from build123d import *

# Parameters (mm, degrees)
CROQUIS1_W              = 56
CROQUIS1_H              = 56
CROQUIS1_R              = 2
SALIENTE_EXTRUIR2_DEPTH = 0.8
CROQUIS4_R              = 4
CROQUIS4_W              = 3.55
CROQUIS4_H              = 40
CORTAR_EXTRUIR1_DEPTH   = 10
CORTAR_EXTRUIR2_START   = -42.374993
CROQUIS7_R              = 2
CORTAR_EXTRUIR2_DEPTH   = 28.749989
SALIENTE_EXTRUIR4_DEPTH = 10


with BuildPart() as part:
    # Croquis1 → Saliente-Extruir2 (new body)
    with BuildSketch(Plane.XY):
        Rectangle(CROQUIS1_W, CROQUIS1_H)
        Circle(CROQUIS1_R, mode=Mode.SUBTRACT)
    extrude(amount=SALIENTE_EXTRUIR2_DEPTH)

    # Croquis2 → Revolución1 (revolve)
    with BuildSketch(Plane(origin=(0, 0, 0), x_dir=(0, 0, -1), z_dir=(1, 0, 0))):
        Polygon((-0.8, 0), (-10.8, 0), (-10.8, 10), (-2.8, 15), (-0.8, 15), align=None)
    revolve(axis=Axis((0, 0, 0.8), (0, 0, 1)))

    # Croquis4 → Cortar-Extruir1 (cut)
    with BuildSketch(Plane.XY.offset(10.8)):
        Circle(CROQUIS4_R)
        with Locations((-6.675, 0)):
            Rectangle(CROQUIS4_W, CROQUIS4_H)
        with Locations((6.675, 0)):
            Rectangle(CROQUIS4_W, CROQUIS4_H)
    extrude(amount=-CORTAR_EXTRUIR1_DEPTH, mode=Mode.SUBTRACT)

    # Croquis7 → Cortar-Extruir2 (cut)
    with BuildSketch(Plane.ZY.offset(28).offset(CORTAR_EXTRUIR2_START)):
        with Locations((5.8, 0)):
            Circle(CROQUIS7_R)
    extrude(amount=CORTAR_EXTRUIR2_DEPTH, mode=Mode.SUBTRACT)

    # Croquis3 → Saliente-Extruir4 (add)
    with BuildSketch(Plane.XY.offset(0.8)):
        with BuildLine():
            Line((23, -28), (28, -28))
            Line((28, -28), (28, -23))
            ThreePointArc((28, -23), (31.535533906, -31.535533906), (23, -28))
        make_face()
    extrude(amount=SALIENTE_EXTRUIR4_DEPTH)


with BuildPart() as saliente_extruir4_kept_piece:
    # of the separate pieces the step leaves, the one the design keeps (saliente_extruir4_pieces_kept)
    add(part.part.solids().sort_by_distance((28, -28, 0))[0])


solid = saliente_extruir4_kept_piece.part
Geometry check sheet. Reference: the model listing, model coordinates, mm. A direction names the side the tool comes from. Round coordinates to 2 decimals unless told otherwise and drop trailing zeros. Write each loop counter-clockwise with the first axis right and the second up, starting at its lowest first coordinate (ties: lowest second). Pieces come first, ordered by that corner, then holes. Notation, with made-up numbers: (-23, -11.5) -> (-2, -11.5) arc R14 ccw to (-2, 14.5) -> close; hole circle Ø2 at (22, -22.75). An arc over 180 degrees is marked (long way). One line per item, written item: value. Start each with the question number.
(1) Draft check along Y on faces 6 (the cylindrical face through (0, 15, 2)), 7 (the cylindrical face through (-0.434, -1.952, 0.394)), 8 (the cylindrical face through (-3.2, -2.4, 5.9)), 9 (the flat face through (-9, 0, 10.8)). Enter one of: +Y half, -Y half, draft (parallel to the pull), parting line (faces both ways), or undercut.
(2) Go/stop test with flat-tipped pins: pin 1 Ø3 at (x, y) = (0, 0) entering from -Z; pin 2 Ø1.5 at (x, y) = (22, -7) entering from +Z; pin 3 Ø4.5 at (y, z) = (0, 5.8) entering from +X; pin 4 Ø5 at (y, z) = (0, 5.8) entering from +X. Record where each tip stops, or that it passes through.
(3) Cross-section at B-B, the plane z = 8.75. Record the cut outline in (x, y).
(4) Scan lines: line 1 (X direction, y = 12, z = 1.75); line 2 (X direction, y = 8, z = 7.25); line 3 (Z direction, x = -4.15, y = 0). Record each from-to range of solid material in increasing order. Write a range as [from, to].
(5) Access from +Z, -Z, +X, -X, +Y, -Y to the whole of each face (thin tool, end or side, straight path). Record for faces 1 (the flat face through (0, 7, 0)), 2 (the cylindrical face through (-15, 0, 2)), 3 (the cylindrical face through (15, 0, 2)), 4 (the flat face through (-8.45, -0.2, 3.6)), 5 (the flat face through (-2, -1, 0.8)).
(6) Cross-section at A-A, the plane x = 0. Record the cut outline in (y, z), and give its area (3 significant figures).
(7) Cross-section at D-D, the plane y = 21. Record the cut outline in (x, z), and give its area (3 significant figures).
(8) Cross-section at C-C, the plane z = 5.8. Record the cut outline in (x, y) (3 decimals), and give its area (3 significant figures).
Answer:
1. face 6: +Y half
1. face 7: undercut
1. face 8: undercut
1. face 9: draft
2. pin 1: through
2. pin 2: z = 0.8
2. pin 3: x = 14.53
2. pin 4: x = 14.69
3. outline: (-8.45, -7.47) -> (-8.45, 7.47) arc R11.28 ccw to start; (-4.9, -10.16) arc R11.28 ccw to (4.9, -10.16) -> (4.9, 10.16) arc R11.28 ccw to (-4.9, 10.16) -> close; (8.45, -7.47) arc R11.28 ccw to (8.45, 7.47) -> close; hole circle Ø8 at (0, 0)
4. line 1: [-9, -8.45], [-4.9, 4.9], [8.45, 9]
4. line 2: [-9.24, -8.45], [-4.9, 4.9], [8.45, 9.24]
4. line 3: [0, 3.8], [7.8, 10.8]
5. face 1: -Z, +X, -X, +Y, -Y
5. face 2: +Z, -X
5. face 3: +Z, +X
5. face 4: +Z, +Y, -Y
5. face 5: +Z
6. outline: (-28, 0) -> (-2, 0) -> (-2, 0.8) -> (-4, 0.8) -> (-4, 10.8) -> (-10, 10.8) -> (-15, 2.8) -> (-15, 0.8) -> (-28, 0.8) -> close; (2, 0) -> (28, 0) -> (28, 0.8) -> (15, 0.8) -> (15, 2.8) -> (10, 10.8) -> (4, 10.8) -> (4, 0.8) -> (2, 0.8) -> close
6. area: 222 mm²
7. outline: (-28, 0) -> (28, 0) -> (28, 0.8) -> (-28, 0.8) -> close
7. area: 44.8 mm²
8. outline: (-12.972, -2) arc R13.125 ccw to (-8.45, -10.043) -> (-8.45, -2) -> close; (-12.972, 2) -> (-8.45, 2) -> (-8.45, 10.043) arc R13.125 ccw to start; (-4.9, -12.176) arc R13.125 ccw to (4.9, -12.176) -> (4.9, -2) -> (3.464, -2) arc R4 cw to (-3.464, -2) -> (-4.9, -2) -> close; (-4.9, 2) -> (-3.464, 2) arc R4 cw to (3.464, 2) -> (4.9, 2) -> (4.9, 12.176) arc R13.125 ccw to (-4.9, 12.176) -> close; (8.45, -10.043) arc R13.125 ccw to (12.972, -2) -> (8.45, -2) -> close; (8.45, 2) -> (12.972, 2) arc R13.125 ccw to (8.45, 10.043) -> close
8. area: 286 mm²
